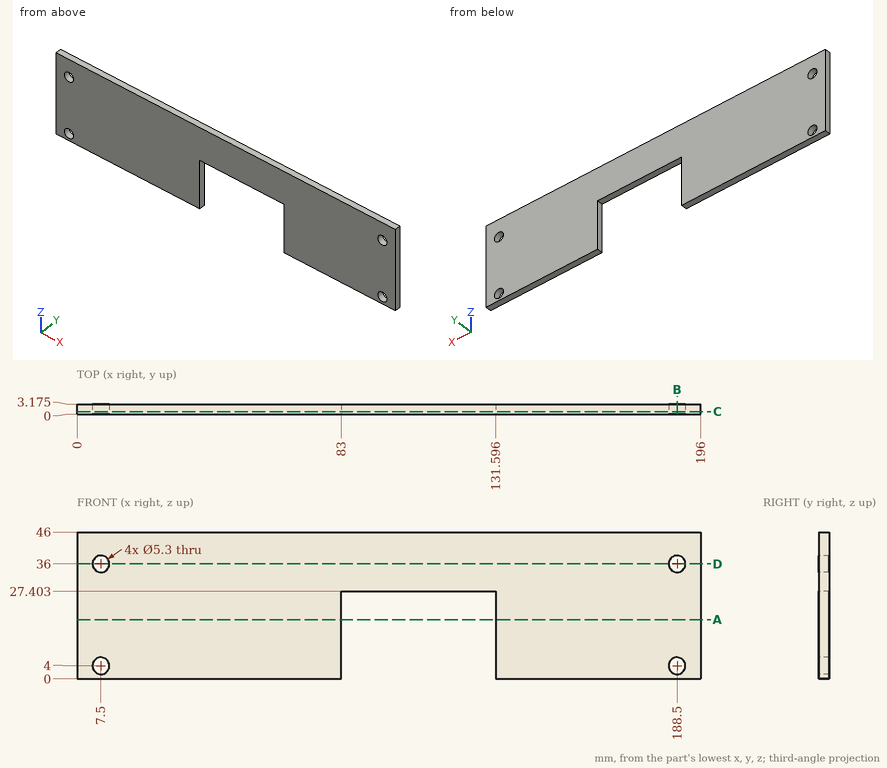
Part print with two shaded views. Sizes in mm from the minimum x, y, z corner. Coordinates: 2 decimals unless noted, no trailing zeros. Order: outer loops, then holes, each group sorted by start corner. A loop starts at its lowest first (then second) coordinate and runs counter-clockwise, first axis right, second up. Notation, with made-up numbers: M 80,-18 L 122,-18 A35 cw 122,16 Z; hole C -30,64 d10. An arc over 180 degrees is marked long. Use a Markdown table: item, result.
(1) Cut at A-A on z = 18.5. Write the cut outline in (x, y) (3 decimals), then the cut area to 3 significant figures.
A:
| item | result |
|---|---|
| outline | M 0,0 L 83,0 L 83,3.175 L 0,3.175 Z; M 131.596,0 L 196,0 L 196,3.175 L 131.596,3.175 Z |
| area | 468 mm^2 |
(2) Probe L1, parallel to Z at x = 188.5, y = 1.6; L2, parallel to X at y = 1, z = 7.5; L3, parallel to Z at x = 95, y = 1.7. List the from-to ranges inside material, lowest first.
A:
| item | result |
|---|---|
| L1 | z = 0 to 1.35, 6.65 to 33.35, 38.65 to 46 |
| L2 | x = 0 to 83, 131.6 to 196 |
| L3 | z = 27.4 to 46 |
(3) Cut at D-D on z = 36. Write the cut outline in (x, y) (3 decimals), then the cut area to 3 significant figures.
A:
| item | result |
|---|---|
| outline | M 0,0 L 4.85,0 L 4.85,3.175 L 0,3.175 Z; M 10.15,0 L 185.85,0 L 185.85,3.175 L 10.15,3.175 Z; M 191.15,0 L 196,0 L 196,3.175 L 191.15,3.175 Z |
| area | 589 mm^2 |
(4) Cut at B-B on x = 188.5. Write the cut outline in (y, z) (3 decimals), then the cut area to 3 significant figures.
A:
| item | result |
|---|---|
| outline | M 0,0 L 3.175,0 L 3.175,1.35 L 0,1.35 Z; M 0,6.65 L 3.175,6.65 L 3.175,33.35 L 0,33.35 Z; M 0,38.65 L 3.175,38.65 L 3.175,46 L 0,46 Z |
| area | 112 mm^2 |
(5) Cut at C-C on y = 0.8. Write the cut outline in (x, z), then the cut area to 3 significant figures.
A:
| item | result |
|---|---|
| outline | M 0,0 L 83,0 L 83,27.4 L 131.6,27.4 L 131.6,0 L 196,0 L 196,46 L 0,46 Z; hole C 7.5,4 d5.3; hole C 7.5,36 d5.3; hole C 188.5,4 d5.3; hole C 188.5,36 d5.3 |
| area | 7,600 mm^2 |
(6) Flat gauge pins, fed straight in: pin 1 (3 mm diameter, centred on x = 7.5, z = 36, fed in from +Y) (1 decimal); pin 2 (1 mm diameter, centred on x = 98, y = 1, fed in from -Z). Where does each tip first touch, or does it go through?
A:
| item | result |
|---|---|
| pin 1 | passes through |
| pin 2 | stops at z = 27.4 |
